Job drawing, mm, ordinate dimensions from the low corner. One solid piece. Give positions to 0.01 mm unless a question says otherwise; leave off trailing zeros. Loops run counter-clockwise (first coordinate to the right, second up) from the corner with the lowest first, then second, coordinate; pieces in that order, holes last. Notation, with made-up numbers: M 50,65 L 105,65 A23 cw 105,96 Z; hole C 51.25,53 d6. An arc over 180 degrees is marked long. Answer in a Markdown table with one row per item.
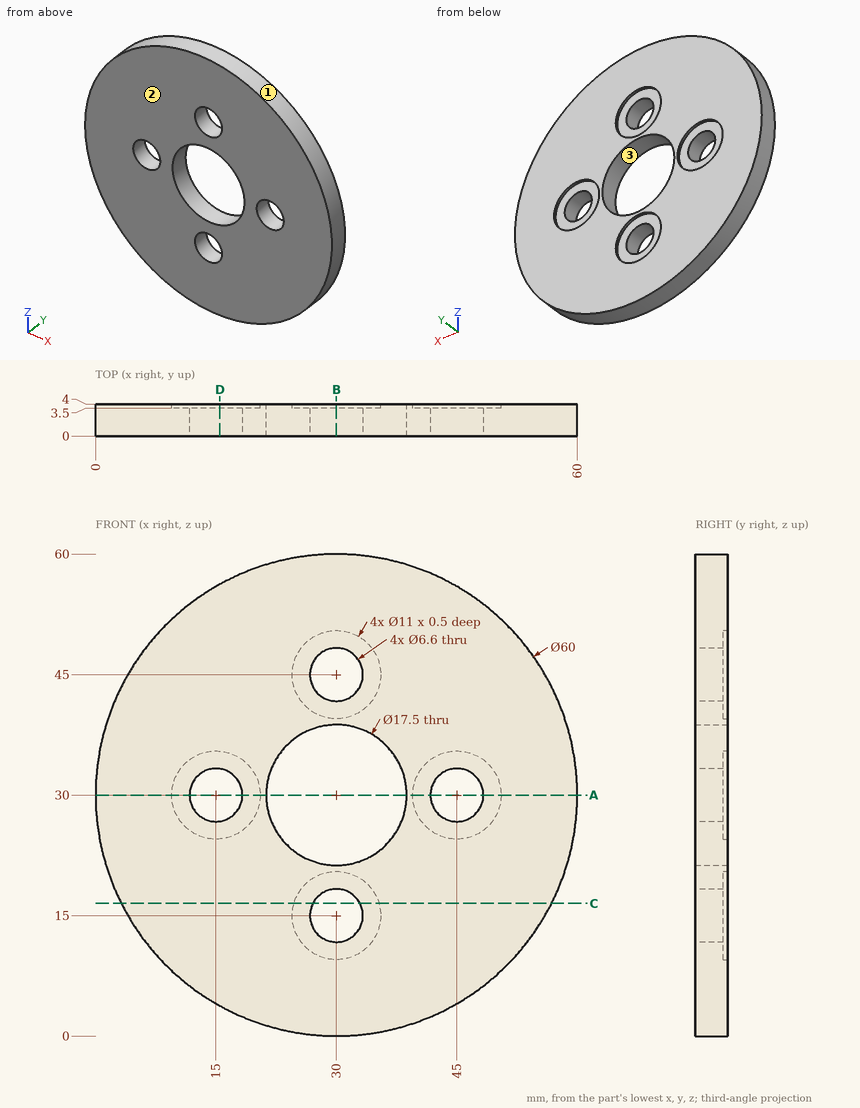
(1) Saw through at C-C (z = 16.5). Write the cut outline in (x, y).
Recorded:
| item | result |
|---|---|
| outline | M 3.21,0 L 27.06,0 L 27.06,3.5 L 24.71,3.5 L 24.71,4 L 3.21,4 Z; M 32.94,0 L 56.79,0 L 56.79,4 L 35.29,4 L 35.29,3.5 L 32.94,3.5 Z |
(2) Pull direction Z, two halves, no side cores. Call the marked faces 1, 2 and 3: +Z half, -Z half, draft (parallel to the pull), parting line (faces both ways), or undercut.
Recorded:
| item | result |
|---|---|
| face 1 | parting line |
| face 2 | draft |
| face 3 | undercut |
(3) Saw through at B-B (x = 30). Write the cut outline in (y, z).
Recorded:
| item | result |
|---|---|
| outline | M 0,0 L 4,0 L 4,9.5 L 3.5,9.5 L 3.5,11.7 L 0,11.7 Z; M 0,18.3 L 3.5,18.3 L 3.5,20.5 L 4,20.5 L 4,21.25 L 0,21.25 Z; M 0,38.75 L 4,38.75 L 4,39.5 L 3.5,39.5 L 3.5,41.7 L 0,41.7 Z; M 0,48.3 L 3.5,48.3 L 3.5,50.5 L 4,50.5 L 4,60 L 0,60 Z |
(4) Pin check, flat tips, straight feed: pin 1 Ø3.5 at (x, z) = (17.5, 30.5) entering from +Y; pin 2 Ø2 at (y, z) = (2, 53) entering from -X; pin 3 Ø3 at (x, z) = (29.5, 49) entering from +Y; pin 4 Ø2 at (x, y) = (51.5, 0.5) entering from +Z. Stop position of each tip, or through.
Recorded:
| item | result |
|---|---|
| pin 1 | stops at y = 3.5 |
| pin 2 | stops at x = 9.6 |
| pin 3 | stops at y = 4 |
| pin 4 | stops at z = 51.9 |
(5) Saw through at D-D (x = 15.5). Write the cut outline in (y, z), plus the area to 3 significant figures.
Recorded:
| item | result |
|---|---|
| outline | M 0,3.74 L 4,3.74 L 4,24.52 L 3.5,24.52 L 3.5,26.74 L 0,26.74 Z; M 0,33.26 L 3.5,33.26 L 3.5,35.48 L 4,35.48 L 4,56.26 L 0,56.26 Z |
| area | 182 mm^2 |
(6) Saw through at A-A (z = 30). Write the cut outline in (x, y).
Recorded:
| item | result |
|---|---|
| outline | M 0,0 L 11.7,0 L 11.7,3.5 L 9.5,3.5 L 9.5,4 L 0,4 Z; M 18.3,0 L 21.25,0 L 21.25,4 L 20.5,4 L 20.5,3.5 L 18.3,3.5 Z; M 38.75,0 L 41.7,0 L 41.7,3.5 L 39.5,3.5 L 39.5,4 L 38.75,4 Z; M 48.3,0 L 60,0 L 60,4 L 50.5,4 L 50.5,3.5 L 48.3,3.5 Z |
(7) Drill centre lines: line 1 along Z through (x, y) = (30, 3.8); line 2 along Z through (x, y) = (30, 2); line 3 along X through (y, z) = (2.85, 29). Where is each one in solid material? Low to high.
Recorded:
| item | result |
|---|---|
| line 1 | z = 0 to 9.5, 20.5 to 21.25, 38.75 to 39.5, 50.5 to 60 |
| line 2 | z = 0 to 11.7, 18.3 to 21.25, 38.75 to 41.7, 48.3 to 60 |
| line 3 | x = 0.02 to 11.86, 18.14 to 21.31, 38.69 to 41.86, 48.14 to 59.98 |
